For this review, take the finished solid that the model builds, in its own axes (mm). Coordinates: 2 decimals unless noted, no trailing zeros. Write each loop counter-clockwise with the first axis right and the second up, starting at its lowest first coordinate (ties: lowest second). Pieces come first, ordered by that corner, then holes. Notation, with made-up numbers: (-24, 20) -> (0, 20) arc R16 cw to (0, 41) -> close; hole circle Ø2 at (-11.75, -3). An arc over 180 degrees is marked (long way). Put each result on its own line as item: value. Start each with the question number.
Item 1: Consider section A-A on z = 15.5. Give the boundary of the cut face in (x, y).
Item 2: To check wall thickness, follow L1, parallel to Z at x = -23, y = 2; L2, parallel to X at y = 2.75, z = 34; L3, parallel to Z at x = -7, y = 5.5. State the ranges of each line that lie inside material, in increasing order.
Item 3: Insertion check: P1, Ø4, axis at x = 8.5, y = 3, coming from the +Z side; P2, Ø11, axis at x = 37.07, z = -24.21, coming from the +Y side; P3, Ø2, axis at x = -33.5, y = 2, coming from the +Z side; P4, Ø1.5, axis at y = 1, z = 18, coming from the +X side. Each pin has a flat end and moves straight along its axis. Give the tip position at first contact, or say it passes through.
Item 4: Consider section B-B on y = 5. Give the boundary of the cut face in (x, z).
Item 5: Consider section C-C on x = 37. Give the boundary of the cut face in (y, z).
```python
from build123d import *
from build123d.topology import SkipClean

# Parameters (mm, degrees)
BOSS_EXTRUDE1_DEPTH = 7
BOSS_EXTRUDE2_DEPTH = 0.5


with BuildPart() as part:
    # Sketch1 → Boss-Extrude1 (new body)
    with BuildSketch(Plane(origin=(0, 0, 0), x_dir=(1, 0, 0), z_dir=(0, 1, 0))):
        with BuildLine():
            Line((29.22824924, 30.681159688), (17.850659856, 16.897054356))
            ThreePointArc((17.850659856, 16.897054356), (15.379675631, 15.1910369), (12.380917697, 15.03705815))
            Line((12.380917697, 15.03705815), (-20.537634361, 17.060906053))
            ThreePointArc((-20.537634361, 17.060906053), (-47.281869491, -27.461627718), (4.525488573, -23.786335009))
            Line((4.525488573, -23.786335009), (17.958953394, 7.231589211))
            ThreePointArc((17.958953394, 7.231589211), (19.505297976, 9.287886756), (21.817685297, 10.415896524))
            Line((21.817685297, 10.415896524), (39.268754989, 14.277407445))
            ThreePointArc((39.268754989, 14.277407445), (45.745634232, 29.516516233), (29.22824924, 30.681159688))
        make_face()
        with BuildLine():
            ThreePointArc((3.607850555, -23.388917762), (-46.445589463, -26.91243355), (-20.537634361, 16.058950924))
            Line((-20.537634361, 16.058950924), (13.195989156, 13.911337267))
            ThreePointArc((13.195989156, 13.911337267), (16.191497408, 14.433261737), (18.621876492, 16.260481579))
            Line((18.621876492, 16.260481579), (29.999465876, 30.044586911))
            ThreePointArc((29.999465876, 30.044586911), (44.89272255, 28.994461003), (39.05270459, 15.253789658))
            Line((39.05270459, 15.253789658), (21.601634898, 11.392278737))
            ThreePointArc((21.601634898, 11.392278737), (18.868813518, 10.059176283), (17.041315376, 7.629006457))
            Line((17.041315376, 7.629006457), (3.607850555, -23.388917762))
        make_face(mode=Mode.SUBTRACT)
    extrude(amount=BOSS_EXTRUDE1_DEPTH)

    # Sketch2 → Boss-Extrude2 (add)
    with SkipClean():  # the faces are left unmerged after this step: merging them gives an invalid solid
        with BuildSketch(Plane(origin=(0, 7, 0), x_dir=(1, 0, 0), z_dir=(0, 1, 0))):
            with BuildLine():
                Line((4.525488573, -23.786335009), (17.958953394, 7.231589211))
                ThreePointArc((17.958953394, 7.231589211), (19.505297976, 9.287886756), (21.817685297, 10.415896524))
                Line((21.817685297, 10.415896524), (39.268754989, 14.277407445))
                ThreePointArc((39.268754989, 14.277407445), (45.745634232, 29.516516233), (29.22824924, 30.681159688))
                Line((29.22824924, 30.681159688), (17.850659856, 16.897054356))
                ThreePointArc((17.850659856, 16.897054356), (15.379675631, 15.1910369), (12.380917697, 15.03705815))
                Line((12.380917697, 15.03705815), (-20.537634361, 17.060906053))
                ThreePointArc((-20.537634361, 17.060906053), (-47.281869491, -27.461627718), (4.525488573, -23.786335009))
            make_face()
            with BuildLine():
                Line((21.601634898, 11.392278737), (39.05270459, 15.253789658))
                ThreePointArc((39.05270459, 15.253789658), (44.89272255, 28.994461003), (29.999465876, 30.044586911))
                Line((29.999465876, 30.044586911), (18.621876492, 16.260481579))
                ThreePointArc((18.621876492, 16.260481579), (16.191497408, 14.433261737), (13.195989156, 13.911337267))
                Line((13.195989156, 13.911337267), (-20.537634361, 16.058950924))
                ThreePointArc((-20.537634361, 16.058950924), (-46.445589463, -26.91243355), (3.607850555, -23.388917762))
                Line((3.607850555, -23.388917762), (17.041315376, 7.629006457))
                ThreePointArc((17.041315376, 7.629006457), (18.868813518, 10.059176283), (21.601634898, 11.392278737))
            make_face(mode=Mode.SUBTRACT)
        extrude(amount=BOSS_EXTRUDE2_DEPTH)


solid = part.part
```
Return value:
1. outline: (-51.41, 0) -> (-50.41, 0) -> (-50.41, 7.5) -> (-51.41, 7.5) -> close; (7.02, 0) -> (8.11, 0) -> (8.11, 7.5) -> (7.02, 7.5) -> close
2. L1: -17.11 to -16.11, 40.42 to 41.42
2. L2: -41.81 to -40.28, -4.39 to -2.85
2. L3: -16.23 to -15.2, 35.9 to 37.09
3. P1: z = 19.23
3. P2: through
3. P3: z = 39.6
3. P4: x = 7.36
4. outline: (-20.54, -17.06) -> (12.38, -15.04) arc R5.5 cw to (17.85, -16.9) -> (29.23, -30.68) arc R10.17 ccw (long way) to (39.27, -14.28) -> (21.82, -10.42) arc R5.5 cw to (17.96, -7.23) -> (4.53, 23.79) arc R29.27 ccw (long way) to start; hole (-20.54, -16.06) -> (13.2, -13.91) arc R6.5 cw to (18.62, -16.26) -> (30, -30.04) arc R9.17 ccw (long way) to (39.05, -15.25) -> (21.6, -11.39) arc R6.5 cw to (17.04, -7.63) -> (3.61, 23.39) arc R28.27 ccw (long way) to start
5. outline: (0, -34.38) -> (7.5, -34.38) -> (7.5, -33.38) -> (0, -33.38) -> close; (0, -14.8) -> (7.5, -14.8) -> (7.5, -13.78) -> (0, -13.78) -> close
